Verification items for the finished model (mm, model axes). A direction names the side the tool comes from. Coordinates: 2 decimals unless noted, no trailing zeros. Loops run counter-clockwise (first coordinate to the right, second up) from the corner with the lowest first, then second, coordinate; pieces in that order, holes last. Notation, with made-up numbers: M 67.25,-28.5 L 105.25,-28.5 A25 cw 105.25,7.5 Z; hole C -30.75,64 d2. An arc over 180 degrees is marked long. Write item = value, one per line. Start each with the question number.
```python
from build123d import *

# Parameters (mm, degrees)
BOX_W           = 55
BOX_H           = 42
BOX_DEPTH       = 17
SKETCH_R        = 1.75
POCKET_DEPTH    = 55.001
POCKET001_DEPTH = 35
POCKET002_DEPTH = 20
SKETCH003_R     = 6.75
POCKET003_DEPTH = 17.001
SKETCH004_R     = 8.25
POCKET004_DEPTH = 7.3
SKETCH005_R     = 8.25
POCKET005_DEPTH = 4.2


with BuildPart() as part:
    # Box → Box (new body)
    with BuildSketch(Plane.XY):
        with Locations((27.5, 21)):
            Rectangle(BOX_W, BOX_H)
    extrude(amount=BOX_DEPTH)

    # Sketch (on Face2 of BaseFeature) → Pocket (cut, through all)
    with BuildSketch(Plane.YZ.offset(55)):
        with Locations((5.5, 13.25)):
            Circle(SKETCH_R)
        with Locations((36.5, 13.25)):
            Circle(SKETCH_R)
    extrude(amount=-POCKET_DEPTH, mode=Mode.SUBTRACT)

    # Sketch001 (on Face2 of BaseFeature) → Pocket001 (cut)
    with BuildSketch(Plane.YZ.offset(55)):
        Polygon((4, 17), (0, 17), (0, 13), align=None)
        Polygon((38, 17), (42, 17), (42, 13), align=None)
    extrude(amount=-POCKET001_DEPTH, mode=Mode.SUBTRACT)

    # Sketch002 (on Face8 of Pocket001) → Pocket002 (cut)
    with BuildSketch(Plane.YZ.offset(55)):
        Polygon((4, 17), (0, 13), (0, 10.5), (3.5, 7), (38.5, 7), (42, 10.5), (42, 13), (38, 17), align=None)
    extrude(amount=-POCKET002_DEPTH, mode=Mode.SUBTRACT)

    # Sketch003 (on Face3 of Pocket002) → Pocket003 (cut, through all)
    with BuildSketch(Plane.XY.offset(17)):
        with Locations((27, 27)):
            Circle(SKETCH003_R)
    extrude(amount=-POCKET003_DEPTH, mode=Mode.SUBTRACT)

    # Sketch004 (on Face3 of Pocket003) → Pocket004 (cut)
    with BuildSketch(Plane.XY.offset(17)):
        with Locations((27, 27)):
            Circle(SKETCH004_R)
    extrude(amount=-POCKET004_DEPTH, mode=Mode.SUBTRACT)

    # Sketch005 (on Face4 of Pocket004) → Pocket005 (cut)
    with BuildSketch(Plane(origin=(0, 0, 0), x_dir=(1, 0, 0), z_dir=(0, 0, -1))):
        with Locations((27, -27)):
            Circle(SKETCH005_R)
    extrude(amount=-POCKET005_DEPTH, mode=Mode.SUBTRACT)


solid = part.part
```
Q1. Set-up check for faces 4 (the face through (20, 40.5, 15.5)), 5 (the face through (45.1, 1.7, 8.8)), 6 (the face through (20, 27, 4.2)), 7 (the face through (28, 2, 15)): record each of +Z, -Z, +X, -X, +Y, -Y from which the full face is reachable in a straight line by a thin tool's end or side.
Q2. Sectioned sample at B-B on x = 27. Record the cut outline in (y, z), plus the area to 3 significant figures.
Q3. Sectioned sample at A-A on y = 5.5. Record the cut outline in (x, z), plus the area to 4 significant figures.
Q4. Scan lines: L1, parallel to Z at x = 7, y = 5.5; L2, parallel to Y at x = 27, z = 13; L3, parallel to Y at x = 27, z = 5.4. Record each from-to range of solid material in increasing order. Write a range as [from, to].
Q5. Sectioned sample at D-D on z = 5.75. Record the cut outline in (x, y).
Q6. Mould release check, pull along X, two halves, no side actions. Record for faces 1 (the face through (22.025, 31.562, 6.988)), 2 (the face through (17.745, 38.169, 13.776)), 3 (the face through (0, 21, 8)): +X half, -X half, draft (parallel to the pull), parting line (faces both ways), or undercut.
Q7. Sectioned sample at C-C on x = 9. Record the cut outline in (y, z), plus the area to 3 significant figures.
Q8. Gauge pin test, flat ends, axial feed: pin 1 (15 mm diameter, centred on x = 27, y = 27, fed in from -Z); pin 2 (5 mm diameter, centred on x = 26, y = 31, fed in from +Z); pin 3 (3 mm diameter, centred on y = 28, z = 14, fed in from +X); pin 4 (1 mm diameter, centred on y = 28, z = 11.5, fed in from +X). Record the tip position at first contact, or that the pin passes through.
Solutions:
q1.face_4 = +Z, +X, +Y
q1.face_5 = +Z, +X
q1.face_6 = -Z
q1.face_7 = +Z, +X, -Y
q2.outline = M 0,0 L 18.75,0 L 18.75,4.2 L 20.25,4.2 L 20.25,9.7 L 18.75,9.7 L 18.75,17 L 4,17 L 0,13 Z; M 33.75,4.2 L 35.25,4.2 L 35.25,0 L 42,0 L 42,13 L 38,17 L 35.25,17 L 35.25,14.47 A1.75 cw long 35.25,12.03 L 35.25,9.7 L 33.75,9.7 Z; hole C 5.5,13.25 d3.5
q2.area = 416 mm²
q3.outline = M 0,0 L 55,0 L 55,7 L 35,7 L 35,11.5 L 0,11.5 Z; M 0,15 L 35,15 L 35,17 L 0,17 Z
q3.area = 612.5 mm²
q4.L1 = [0, 11.5], [15, 17]
q4.L2 = [0, 3.77], [7.23, 18.75], [38.23, 42]
q4.L3 = [0, 20.25], [33.75, 42]
q5.outline = M 0,0 L 55,0 L 55,42 L 0,42 Z; hole C 27,27 d13.5
q6.face_1 = undercut
q6.face_2 = draft
q6.face_3 = -X half
q7.outline = M 0,0 L 42,0 L 42,17 L 0,17 Z; hole C 5.5,13.25 d3.5; hole C 36.5,13.25 d3.5
q7.area = 695 mm²
q8.pin_1 = 4.2
q8.pin_2 = through
q8.pin_3 = 35
q8.pin_4 = 18.89
